Source: CAD feature listing. Evaluate the final solid. Frame: model axes, mm. Give positions to 0.01 mm unless a question says otherwise; leave off trailing zeros. Order: outer loops, then holes, each group sorted by start corner. A loop starts at its lowest first (then second) coordinate and runs counter-clockwise, first axis right, second up.
1) Section C-C, the plane z = -489. Return loops of the section in (x, y) (3 decimals), plus the area to 3 significant figures.
2) Material intervals for line 1 (Z direction, x = 521, y = 2.5); line 2 (X direction, y = 5.75, z = -545); line 3 (X direction, y = 4.25, z = -491), sorted ascending.
3) Section B-B, the plane x = 460.5. Return loops of the section in (y, z) (3 decimals).
4) Section A-A, the plane y = 6.75. Return loops of the section in (x, z).
```python
from build123d import *

# Parameters (mm, degrees)
SKETCH1_W            = 1219.2
SKETCH1_H            = 1219.2
BOSS_EXTRUDE1_DEPTH  = 9.525
CUT_EXTRUDE1_REACH   = 864.157
SKETCH2_R            = 152.4
CUT_EXTRUDE2_DEPTH   = 863.157204705
MIRROR2_COPY_1_DEPTH = 863.157204705
FILLET1_R            = 50.8


with BuildPart() as part:
    # Sketch1 → Boss-Extrude1 (new body)
    with BuildSketch(Plane(origin=(0, 0, 0), x_dir=(1, 0, 0), z_dir=(0, 1, 0))):
        Rectangle(SKETCH1_W, SKETCH1_H)
    extrude(amount=BOSS_EXTRUDE1_DEPTH)

    # Sketch2 → Cut-Extrude1 (cut, up to next)
    with BuildSketch(Plane(origin=(0, 9.525, 0), x_dir=(1, 0, 0), z_dir=(0, 1, 0)), mode=Mode.PRIVATE) as cut_extrude1_sk1:
        with Locations((-609.6, 609.6)):
            Circle(SKETCH2_R)
    cut_extrude1_tool1 = extrude(cut_extrude1_sk1.sketch, amount=-CUT_EXTRUDE1_REACH, mode=Mode.PRIVATE) & part.part
    # Sketch2 → Cut-Extrude1 (cut, up to next)
    with BuildSketch(Plane(origin=(0, 9.525, 0), x_dir=(1, 0, 0), z_dir=(0, 1, 0)), mode=Mode.PRIVATE) as cut_extrude1_sk2:
        with Locations((-609.6, -609.6)):
            Circle(SKETCH2_R)
    cut_extrude1_tool2 = extrude(cut_extrude1_sk2.sketch, amount=-CUT_EXTRUDE1_REACH, mode=Mode.PRIVATE) & part.part
    # Sketch2 → Cut-Extrude1 (cut, up to next)
    with BuildSketch(Plane(origin=(0, 9.525, 0), x_dir=(1, 0, 0), z_dir=(0, 1, 0)), mode=Mode.PRIVATE) as cut_extrude1_sk3:
        with Locations((609.6, -609.6)):
            Circle(SKETCH2_R)
    cut_extrude1_tool3 = extrude(cut_extrude1_sk3.sketch, amount=-CUT_EXTRUDE1_REACH, mode=Mode.PRIVATE) & part.part
    # Sketch2 → Cut-Extrude1 (cut, up to next)
    with BuildSketch(Plane(origin=(0, 9.525, 0), x_dir=(1, 0, 0), z_dir=(0, 1, 0)), mode=Mode.PRIVATE) as cut_extrude1_sk4:
        with Locations((609.6, 609.6)):
            Circle(SKETCH2_R)
    cut_extrude1_tool4 = extrude(cut_extrude1_sk4.sketch, amount=-CUT_EXTRUDE1_REACH, mode=Mode.PRIVATE) & part.part
    add(cut_extrude1_tool1.solids().sort_by_distance((-609.6, 9.525, -609.6))[0], mode=Mode.SUBTRACT)
    add(cut_extrude1_tool2.solids().sort_by_distance((-609.6, 9.525, 609.6))[0], mode=Mode.SUBTRACT)
    add(cut_extrude1_tool3.solids().sort_by_distance((609.6, 9.525, 609.6))[0], mode=Mode.SUBTRACT)
    add(cut_extrude1_tool4.solids().sort_by_distance((609.6, 9.525, -609.6))[0], mode=Mode.SUBTRACT)

    # Sketch3 → Cut-Extrude2 (cut, symmetric)
    with BuildSketch(Plane(origin=(0, 9.525, 0), x_dir=(1, 0, 0), z_dir=(0, 1, 0))):
        Polygon((-1846.295154261, 2849.969007356), (394.073853094, 609.6), (609.6, 394.073853094), (2849.969007356, -1846.295154261), (7330.707022067, 2634.44286045), (2634.44286045, 7330.707022067), align=None)
    cut_extrude2 = extrude(amount=CUT_EXTRUDE2_DEPTH, both=True, mode=Mode.SUBTRACT)

    # Mirror1: Cut-Extrude2 across plane
    add(cut_extrude2.mirror(Plane.XY), mode=Mode.SUBTRACT)

    # Mirror2: Cut-Extrude2 across plane
    add(cut_extrude2.mirror(Plane(origin=(0, 0, 0), x_dir=(0, 0, 1), z_dir=(1, 0, 0))), mode=Mode.SUBTRACT)

    # Mirror2 copy 1 sketch → Mirror2 copy 1 (cut, symmetric)
    with BuildSketch(Plane(origin=(0, 9.525, 0), x_dir=(-1, 0, 0), z_dir=(0, 1, 0))):
        Polygon((-1846.295154261, 2849.969007356), (394.073853094, 609.6), (609.6, 394.073853094), (2849.969007356, -1846.295154261), (7330.707022067, 2634.44286045), (2634.44286045, 7330.707022067), align=None)
    extrude(amount=MIRROR2_COPY_1_DEPTH, both=True, mode=Mode.SUBTRACT)

    # Fillet1
    fillet1_edges = [part.edges().sort_by_distance(p)[0] for p in [
        (-609.6, 4.7625, -394.073853094),
        (-394.073853094, 4.7625, -609.6),
        (-609.6, 4.7625, 394.073853094),
        (-394.073853094, 4.7625, 609.6),
        (609.6, 4.7625, -394.073853094),
        (394.073853094, 4.7625, -609.6),
        (609.6, 4.7625, 394.073853094),
        (394.073853094, 4.7625, 609.6),
    ]]
    fillet(fillet1_edges, radius=FILLET1_R)


solid = part.part
```
From the geometry:
1. outline: (-514.674, 0) - (514.674, 0) - (514.674, 9.525) - (-514.674, 9.525) - close
1. area: 9,800 mm2
2. line 1: z = -482.67 to 482.67
2. line 2: x = -458.67 to 458.67
2. line 3: x = -512.67 to 512.67
3. outline: (0, -543.174) - (9.525, -543.174) - (9.525, 543.174) - (0, 543.174) - close
4. outline: (-609.6, -373.03) arc R50.8 ccw to (-594.72, -408.95) - (-408.95, -594.72) arc R50.8 ccw to (-373.03, -609.6) - (373.03, -609.6) arc R50.8 ccw to (408.95, -594.72) - (594.72, -408.95) arc R50.8 ccw to (609.6, -373.03) - (609.6, 373.03) arc R50.8 ccw to (594.72, 408.95) - (408.95, 594.72) arc R50.8 ccw to (373.03, 609.6) - (-373.03, 609.6) arc R50.8 ccw to (-408.95, 594.72) - (-594.72, 408.95) arc R50.8 ccw to (-609.6, 373.03) - close
